Autodesk Inventor part; units mm, degrees
ref_plane "YZ Plane" through (0, 0, 0) normal (1, 0, 0) x (0, 1, 0)
ref_plane "XZ Plane" through (0, 0, 0) normal (0, 1, 0) x (-1, 0, 0)
ref_plane "XY Plane" through (0, 0, 0) normal (0, 0, 1) x (1, 0, 0)
sketch "Sketch1" plane through (0, 0, 0) normal (0, 1, 0) x (-1, 0, 0)
  line L0 (85, 30) -> (-85, 30)
  line L1 (-85, 30) -> (-85, -30)
  line L2 (-85, -30) -> (85, -30)
  line L3 (85, -30) -> (85, 30)
  line L4 (85, 30) -> (-85, -30) construction
  line L5 (-85, 30) -> (85, -30) construction
  line L6 (0, -42) -> (0, 42)
  point P0 (0, 0)
  point P1 (-100, -30)
  point P2 (-85, -27)
  dimension "d0" = 170
  dimension "d1" = 60
  dimension "d32" = 15
extrude "Extrusion1" add sketch "Sketch1" along normal blind 3
sketch "Sketch2" plane through (0, 3, 0) normal (0, 1, 0) x (1, 0, 0)
  line L0 (-85, 30) -> (-85, -30)
  line L1 (-85, -30) -> (85, -30)
  line L2 (85, -30) -> (85, 30)
  line L3 (80, -25) -> (-80, -25)
  line L4 (-80, -25) -> (-80, 25)
  line L5 (-80, 25) -> (80, 25)
  line L6 (80, 25) -> (80, -25)
  line L7 (80, -25) -> (-80, 25) construction
  line L8 (-80, -25) -> (80, 25) construction
  line L9 (85, 30) -> (-85, 30)
  point P0 (0, 0)
  dimension "d36" = 160
  dimension "d37" = 50
extrude "Extrusion2" add sketch "Sketch2" along normal blind 28
sketch "Sketch7" plane through (-80, 3, 25) normal (1, 0, 0) x (0, 0, -1)
  circle A0 centre (10, 14) radius 8
  line L0 (55, -3) -> (-5, -3)
  circle A1 centre (10, 14) radius 10
  line L1 (0, 14) -> (0, 0)
  line L2 (0, 14) -> (20, 14)
  line L3 (20, 14) -> (20, 0)
  line L4 (-5, -3) -> (-5, 28)
  line L5 (0, 0) -> (20, 0)
  line L6 (10, 24) -> (0, 24)
  line L7 (0, 0) -> (0, 28)
  line L8 (0, 14) -> (0, 24)
  point P0 (25, -3)
  point P1 (54, -3)
  dimension "MotorDiameter" = 16
  dimension "d18" = 17
  dimension "d20" = 2
  dimension "d40" = 20
  dimension "d62" = 10
extrude "Extrusion5" add sketch "Sketch7" along normal blind 11.25 contours L2 A1 A0 | A0 L2 A1 | L3 L5 L1 A1 | L7 L6 A1
sketch "Sketch8" plane through (-68.75, 3, 25) normal (1, 0, 0) x (0, 0, -1)
  arc A0 (20, 14) -> (10, 24) centre (10, 14) ccw
  circle A1 centre (10, 14) radius 8
  line L0 (0, 0) -> (0, 24)
  line L1 (20, 0) -> (0, 0)
  line L2 (20, 0) -> (20, 14)
  circle A2 centre (10, 14) radius 7.75
  line L3 (10, 24) -> (0, 24)
  line L4 (0, 0) -> (0, 24)
  line L5 (4, 9.0946) -> (4, 19.2915)
  line L6 (10, 24) -> (0, 24)
  line L7 (16, 9.0946) -> (16, 19.2915)
  line L8 (16, 19.2915) -> (18.4853, 19.2915)
  arc A3 (20, 14) -> (10, 24) centre (10, 14) ccw
  line L9 (4, 19.2915) -> (0, 19.2915)
  point P0 (25, -3)
  point P1 (4, 27)
  point P2 (4, 18.9054)
  point P3 (16, 18.9054)
  dimension "d55" = 15.5
  dimension "d63" = 12
  dimension "d64" = 6
extrude "Extrusion6" add sketch "Sketch8" along normal blind 20 contours L2 L1 L0 L9 A1 L8 A0 | A1 L5 A2 L7 | A2 L7 | L5 A2 picked at (9.114, 6.2488)
sketch "Sketch9" plane through (-80, 20, 19) normal (1, 0, 0) x (0, 0, -1)
  circle A0 centre (4, -3) radius 3.5
  line L0 (49, -20) -> (-11, -20)
  line L1 (-11, -20) -> (-11, 11)
  point P0 (19, -20)
  point P1 (44, -20)
  dimension "d27" = 7
  dimension "d28" = 17
  dimension "d41" = 15
extrude "Extrusion7" cut sketch "Sketch9" against normal up to surface (5 mm away)
mirror "Mirror2" about plane through (0, 0, 0) normal (1, 0, 0) of "Extrusion7", "Extrusion6", "Extrusion5"
sketch "Sketch14" plane through (0, 3, 0) normal (0, 1, 0) x (1, 0, 0)
  point P0 (0, 0)
sketch "Sketch15" plane through (85, 0, 30) normal (1, 0, 0) x (0, 0, -1)
  line L0 (60, 31) -> (0, 31)
  line L1 (60, 31) -> (120, 0)
  line L2 (120, 0) -> (60, 0)
  circle A0 centre (15, 17) radius 3.5
  line L3 (0, 0) -> (60, 0)
  line L4 (60, 0) -> (60, 31)
  line L5 (0, 31) -> (60, 31)
  line L6 (0, 0) -> (0, 31)
  point P0 (30, 0)
  dimension "d67" = 60
extrude "Extrusion12" add sketch "Sketch15" against normal blind 3 contours L1 L2 L4
mirror "Mirror5" about plane through (0, 0, 0) normal (1, 0, 0) of "Extrusion12"
equation "\"d0\" = Width"
equation "\"d1\" = Length"
equation "\"d2\" = BaseWallThickness"
equation "\"d36\" = Width - 2 * SideWallThickness"
equation "\"d37\" = Length - 2 * SideWallThickness"
equation "\"d5\" = Height - 2 * BaseWallThickness"
equation "\"d18\" = DriveMotorHeight"
equation "\"d20\" = DriveMotorMountThickness"
equation "\"d28\" = DriveMotorHeight"
equation "\"d41\" = SideWallThickness + DriveMotorMountThickness + 0.5 * MotorDiameter"
equation "\"d67\" = WedgeLength"
equation "\"d68\" = BaseWallThickness"
equation "\"SideWallThickness\" = 5"
equation "\"BaseWallThickness\" = 3"
equation "\"Width\" = 170"
equation "\"Length\" = 60"
equation "\"Height\" = 34"
equation "\"DriveMotorHeight\" = 17"
equation "\"DriveMotorMountThickness\" = 2"
equation "\"WedgeLength\" = 60"
properties part number "BodyWedgeV1" material "Thermoplastic Resin"
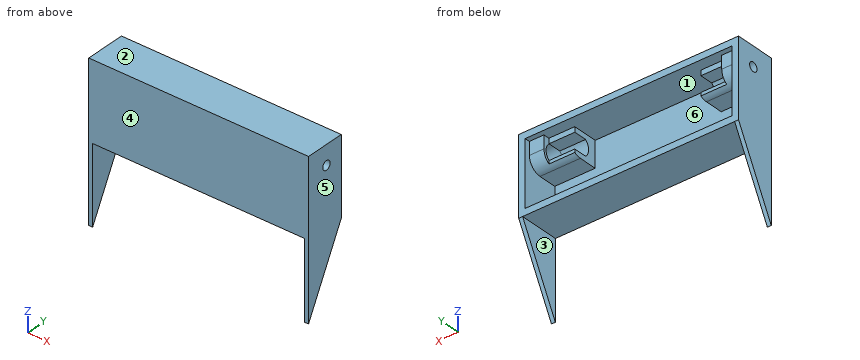
CAD build for the part. Positions are in the model's coordinates, mm. Face numbers are marked on the shaded views. A direction names the side the tool comes from. Round coordinates to 2 decimals unless told otherwise and drop trailing zeros. Loops run counter-clockwise (first coordinate to the right, second up) from the corner with the lowest first, then second, coordinate; pieces in that order, holes last. Notation, with made-up numbers: M -36.75,-24.5 L 2.25,-24.5 A24 ccw 2.25,10.5 Z; hole C 81.5,-15 d2. An arc over 180 degrees is marked long. One line per question, with ' | ' between items. Start each with the question number.
Item 1: Which spindle directions (+Z, -Z, +X, -X, +Y, -Y) get a long thin tool onto all of the face, cutting with end or side? Do the marked faces 1, 2 and 3. Say none if no direction does.
Item 2: Two-plate mould, pull along X, no slides. Class the marked faces 4, 5 and 6: pulls with the +X half, pulls with the -X half, needs draft (parallel to the pull), parting line crosses it, or undercut.
Item 3: Cut at B-B, the plane x = 71.5. Write the cut outline in (y, z), plus the area to 3 significant figures.
Item 4: Pin check, flat tips, straight feed: pin 1 Ø6.5 at (y, z) = (17, 15) entering from +X; pin 2 Ø2 at (x, z) = (-58.5, 7.5) entering from +Y; pin 3 Ø5 at (x, z) = (-73, 20) entering from +Y; pin 4 Ø7 at (x, y) = (57.5, 10.5) entering from -Z. Stop position of each tip, or through.
Item 5: Cut at D-D, the plane z = 2. Write the cut outline in (x, y).
Item 6: Cut at A-A, the plane z = -42. Write the cut outline in (x, y).
Item 7: Cut at C-C, the plane x = 9. Write the cut outline in (y, z).
Item 8: Wall check: line 1 (Z direction, x = 51.5, y = 17); line 2 (Z direction, x = 71.5, y = 17); line 3 (Y direction, x = -76, z = 15). Give the ranges that are in metal, low to high.
Responses:
1) face 1: +Y | face 2: +Z, +X, -X, +Y, -Y | face 3: -Z, +Y, -Y
2) face 4: needs draft | face 5: pulls with the +X half | face 6: undercut
3) outline: M 0,-30 L 31,-30 L 31,-25 L 3,-25 L 3,5 L 17,5 A10 ccw 27,15 L 27,25 L 31,25 L 31,30 L 0,30 Z; hole C 17,15 d16 | area: 717 mm²
4) pin 1: passes through | pin 2: stops at y = 22.29 | pin 3: stops at y = 27 | pin 4: stops at z = -30
5) outline: M -85,0 L 85,0 L 85,31 L 80,31 L 80,3 L -80,3 L -80,31 L -85,31 Z
6) outline: M -85,0 L -82,0 L -82,24.8 L -85,24.8 Z; M 82,0 L 85,0 L 85,24.8 L 82,24.8 Z
7) outline: M 0,-30 L 31,-30 L 31,-25 L 3,-25 L 3,25 L 31,25 L 31,30 L 0,30 Z
8) line 1: z = -30 to -25, 5 to 9, 21 to 30 | line 2: z = -30 to -25, 5 to 7, 23 to 30 | line 3: y = 0 to 9, 25 to 27
